Geometry check sheet. Reference: the model listing, model coordinates, mm. Coordinates: 2 decimals unless noted, no trailing zeros. Order: outer loops, then holes, each group sorted by start corner. A loop starts at its lowest first (then second) coordinate and runs counter-clockwise, first axis right, second up. Notation, with made-up numbers: (75, 46) - (84, 46) arc R13 ccw to (84, 61) - close; hole circle Ø8 at (49, -3.75). An arc over 180 degrees is marked (long way). One line per item, written item: value. Start each with the question number.
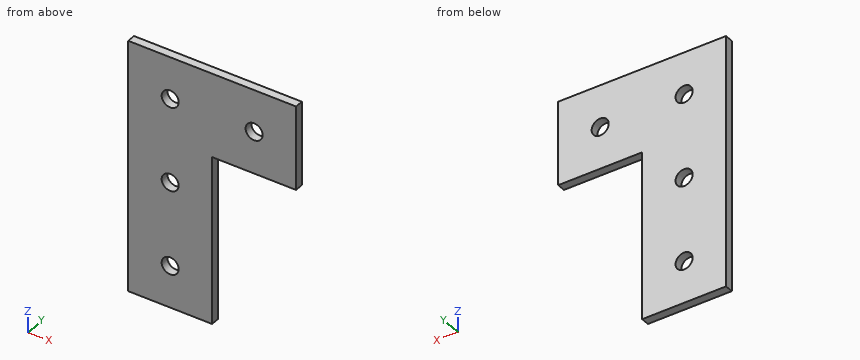
Autodesk Inventor part; units mm, degrees
ref_plane "YZ Plane" through (0, 0, 0) normal (1, 0, 0) x (0, 1, 0)
ref_plane "XZ Plane" through (0, 0, 0) normal (0, 1, 0) x (-1, 0, 0)
ref_plane "XY Plane" through (0, 0, 0) normal (0, 0, 1) x (1, 0, 0)
sketch "Sketch1" plane through (0, 0, 0) normal (0, 1, 0) x (-1, 0, 0)
  line L0 (0, 0) -> (-25.4, 0)
  line L1 (-25.4, 0) -> (-25.4, 76.2)
  line L2 (-25.4, 76.2) -> (0, 76.2)
  line L3 (0, 76.2) -> (0, 0)
  line L4 (-25.4, 76.2) -> (-50.8, 76.2)
  line L5 (-50.8, 76.2) -> (-50.8, 50.8)
  line L6 (-50.8, 50.8) -> (-25.4, 50.8)
  line L7 (-25.4, 50.8) -> (-25.4, 76.2)
  circle A0 centre (-12.7, 12.7) radius 2.5797
  circle A1 centre (-38.1, 63.5) radius 2.5797
  circle A2 centre (-12.7, 38.1) radius 2.5797
  circle A3 centre (-12.7, 63.5) radius 2.5797
  dimension "d0" = 76.2
  dimension "d1" = 25.4
  dimension "d2" = 25.4
  dimension "d3" = 25.4
  dimension "d5" = 38.1
  dimension "d7" = 25.4
  dimension "d8" = 25.4
  dimension "d11" = 12.7
  dimension "d12" = 12.7
  dimension "d13" = 12.7
  dimension "d14" = 5.1594
  dimension "d15" = 5.1594
  dimension "d16" = 5.1594
  dimension "d17" = 5.1594
  dimension "d18" = 12.7
  dimension "d19" = 25.4
  dimension "d20" = 12.7
extrude "Extrusion1" add sketch "Sketch1" along normal blind 2.54
equation "\"d15\" = d14"
equation "\"d16\" = d14"
equation "\"d17\" = d14"
properties part number "bracing 2x3"
Q1. Cross-section at B-B, the plane z = 63.5. Enter the section's corners in (x, y).
Q2. Material ranges on probe 1 along Z at (x, y) = (12.7, 1.55); probe 2 along Z at (x, y) = (38, 2.45); probe 3 along X at (y, z) = (2.4, 64), recorded low to high.
Q3. Cross-section at C-C, the plane z = 12.7. Enter the section's corners in (x, y), and give its area (3 significant figures).
Q4. Gauge pin test, flat end, axial feed: P1, Ø1.3, axis at y = 2, z = 22.5, coming from the +X side. Record the tip position at first contact, or that the pin passes through.
Q5. Cross-section at A-A, the plane x = 12.7. Enter the section's corners in (y, z), and give its area (3 significant figures).
Q6. Cross-section at D-D, the plane y = 1.05. Enter the section's corners in (x, z).
Check result:
1. outline: (0, 0) - (10.12, 0) - (10.12, 2.54) - (0, 2.54) - close; (15.28, 0) - (35.52, 0) - (35.52, 2.54) - (15.28, 2.54) - close; (40.68, 0) - (50.8, 0) - (50.8, 2.54) - (40.68, 2.54) - close
2. probe 1: z = 0 to 10.12, 15.28 to 35.52, 40.68 to 60.92, 66.08 to 76.2
2. probe 2: z = 50.8 to 60.92, 66.08 to 76.2
2. probe 3: x = 0 to 10.17, 15.23 to 35.57, 40.63 to 50.8
3. outline: (0, 0) - (10.12, 0) - (10.12, 2.54) - (0, 2.54) - close; (15.28, 0) - (25.4, 0) - (25.4, 2.54) - (15.28, 2.54) - close
3. area: 51.4 mm2
4. P1: stops at x = 25.4
5. outline: (0, 0) - (2.54, 0) - (2.54, 10.12) - (0, 10.12) - close; (0, 15.28) - (2.54, 15.28) - (2.54, 35.52) - (0, 35.52) - close; (0, 40.68) - (2.54, 40.68) - (2.54, 60.92) - (0, 60.92) - close; (0, 66.08) - (2.54, 66.08) - (2.54, 76.2) - (0, 76.2) - close
5. area: 154 mm2
6. outline: (0, 0) - (25.4, 0) - (25.4, 50.8) - (50.8, 50.8) - (50.8, 76.2) - (0, 76.2) - close; hole circle Ø5.16 at (12.7, 12.7); hole circle Ø5.16 at (12.7, 38.1); hole circle Ø5.16 at (12.7, 63.5); hole circle Ø5.16 at (38.1, 63.5)
